Can you work these out from the model? Positions are in its coordinate system, mm. Face numbers are marked on the shaded views. A direction names the side the tool comes from. Give positions to 0.01 mm unless a question says otherwise; leave off trailing zeros. Loops run counter-clockwise (first coordinate to the right, second up) from the corner with the lowest first, then second, coordinate; pieces in that order, holes last. Notation, with made-up numbers: M 44.5,39 L 103.5,39 A12 cw 103.5,56 Z; hole C 62.25,66.25 d4. An arc over 180 degrees is marked long. Use CSV: the item, a comma, the result in double quotes.
from build123d import *

# Parameters (mm, degrees)
F1_DEPTH = 36
F3_D     = 5.5
F3_DEPTH = 10
F3_TIP   = 1.6523667023
F5_R     = 17.5
F6_DEPTH = 59
F7_R     = 8
F8_DEPTH = 95.001
F10_D    = 21


with BuildPart() as f1:
    # F0 (on Top) → F1 (new body)
    with BuildSketch(Plane.XY):
        with BuildLine():
            Line((19.6214168703, 36), (-19.6214168703, 36))
            ThreePointArc((-19.6214168703, 36), (-28.9913780286, 28.9913780286), (-36, 19.6214168703))
            Line((-36, 19.6214168703), (-36, -19.6214168703))
            ThreePointArc((-36, -19.6214168703), (-28.9913780286, -28.9913780286), (-19.6214168703, -36))
            Line((-19.6214168703, -36), (19.6214168703, -36))
            ThreePointArc((19.6214168703, -36), (28.9913780286, -28.9913780286), (36, -19.6214168703))
            Line((36, -19.6214168703), (36, 19.6214168703))
            ThreePointArc((36, 19.6214168703), (28.9913780286, 28.9913780286), (19.6214168703, 36))
        make_face()
    extrude(amount=F1_DEPTH)

    # F3
    with Locations(Plane.XY.offset(36)):
        with Locations((-24.7487373415, 24.7487373415), (24.7487373415, 24.7487373415), (24.7487373415, -24.7487373415), (-24.7487373415, -24.7487373415)):
            Hole(F3_D / 2, depth=F3_DEPTH)
            with Locations((0, 0, -(F3_DEPTH + F3_TIP / 2))):  # 118° drill point
                Cone(0, F3_D / 2, F3_TIP, mode=Mode.SUBTRACT)

    # F5 (on face) → F6 (join)
    with BuildSketch(Plane(origin=(0, 0, 0), x_dir=(1, 0, 0), z_dir=(0, 0, -1))):
        Circle(F5_R)
    extrude(amount=F6_DEPTH)

    # F7 (on face) → F8 (cut, through all)
    with BuildSketch(Plane(origin=(0, 0, -59), x_dir=(1, 0, 0), z_dir=(0, 0, -1))):
        Circle(F7_R)
    extrude(amount=-F8_DEPTH, mode=Mode.SUBTRACT)

    # F10 (through all)
    with Locations(Plane(origin=(0, 36, 0), x_dir=(-1, 0, 0), z_dir=(0, 1, 0))):
        with Locations((0, 18)):
            Hole(F10_D / 2)


solid = f1.part
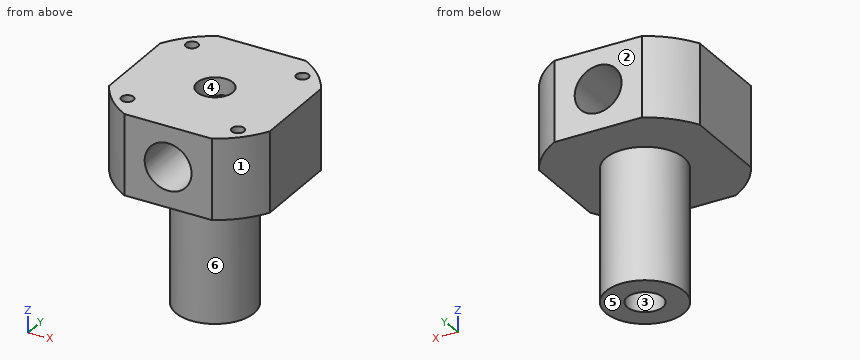
Q1. If we mould it in two halves opening along X, with no side actions, what happens to the marked faces 1, 2, 3 and 4? For each: released by +X, released by -X, zero draft, split by the parting line, or undercut.
Model answer:
face 1,"released by +X"
face 2,"zero draft"
face 3,"undercut"
face 4,"undercut"
Q2. I want a section at B-B, the plane x = 0. Please give me the cut outline in (y, z), then the cut area to 3 significant figures.
Model answer:
outline,"M -36,0 L -17.5,0 L -17.5,-59 L -8,-59 L -8,7.5 L -36,7.5 Z; M -36,28.5 L -8,28.5 L -8,36 L -36,36 Z; M 8,-59 L 17.5,-59 L 17.5,0 L 36,0 L 36,7.5 L 8,7.5 Z; M 8,28.5 L 36,28.5 L 36,36 L 8,36 Z"
area,"1,960 mm2"
Q3. For the marked faces 5 and 6, which set-ups out of +Z, -Z, +X, -X, +Y, -Y let a thin tool reach every point of the face, with its end or its side?
Model answer:
face 5,"-Z, +X, -X, +Y, -Y"
face 6,"-Z"
Q4. I want a section at A-A, the plane z = 18. Please give me the cut outline in (x, y), then the cut area to 3 significant figures.
Model answer:
outline,"M -36,-19.62 A41 ccw -19.62,-36 L -10.5,-36 L -10.5,36 L -19.62,36 A41 ccw -36,19.62 Z; M 10.5,-36 L 19.62,-36 A41 ccw 36,-19.62 L 36,19.62 A41 ccw 19.62,36 L 10.5,36 Z"
area,"3,240 mm2"
Q5. I want a section at C-C, the plane y = 0. Please give me the cut outline in (x, z), then the cut area to 3 significant figures.
Model answer:
outline,"M -36,0 L -17.5,0 L -17.5,-59 L -8,-59 L -8,11.2 A10.5 cw -8,24.8 L -8,36 L -36,36 Z; M 8,-59 L 17.5,-59 L 17.5,0 L 36,0 L 36,36 L 8,36 L 8,24.8 A10.5 cw 8,11.2 Z"
area,"3,090 mm2"
Q6. Please list where these lines run through material, in increasing order: L1, parallel to Z at x = 0, y = 21; L2, parallel to X at y = 0, z = 28. Write a range as from..to.
Model answer:
L1,"0..7.5, 28.5..36"
L2,"-36..-8, 8..36"
Q7. I'm going to push flat-ended pins straight in: P1, Ø4.5, axis at x = -24.75, y = -24.75, coming from the +Z side; P2, Ø12, axis at x = -27.5, y = 2.5, coming from the -Z side; P3, Ø1, axis at x = 28, z = 24.5, coming from the -Y side. Where does each tip first touch, or does it pass through?
Model answer:
P1,"z = 25.7"
P2,"z = 0"
P3,"y = -30.41"
Q8. I want a section at D-D, the plane y = 10.5. Please give me the cut outline in (x, z).
Model answer:
outline,"M -36,0 L -14,0 L -14,-59 L 14,-59 L 14,0 L 36,0 L 36,36 L -36,36 Z; hole C 0,18 d21"
